```python
from build123d import *

# Parameters (mm, degrees)
SKETCH1_W           = 80
SKETCH1_H           = 80
BOSS_EXTRUDE3_DEPTH = 2
BOSS_EXTRUDE5_DEPTH = 77.35
CUT_EXTRUDE1_REACH  = 58.918
SKETCH7_W           = 64.6
SKETCH7_H           = 77
SKETCH5_W           = 80
SKETCH5_H           = 80
SKETCH5_W_2         = 77
SKETCH5_H_2         = 77
BOSS_EXTRUDE6_DEPTH = 44.8
SKETCH8_W           = 80
SKETCH8_H           = 80
BOSS_EXTRUDE7_DEPTH = 1.5


with BuildPart() as part:
    # Sketch1 → Boss-Extrude3 (new body)
    with BuildSketch(Plane(origin=(0, 0, 0), x_dir=(1, 0, 0), z_dir=(0, 1, 0))):
        Rectangle(SKETCH1_W, SKETCH1_H)
    extrude(amount=-BOSS_EXTRUDE3_DEPTH)

    # Sketch3 → Boss-Extrude5 (add)
    with BuildSketch(Plane.XY.offset(40)):
        Polygon((-32.3, -2), (-34.8, -2), (-34.8, -4.3), (-37.3, -4.3), (-37.3, -6.3), (-32.3, -6.3), align=None)
        Polygon((32.3, -6.3), (37.3, -6.3), (37.3, -4.3), (34.8, -4.3), (34.8, -2), (32.3, -2), align=None)
    extrude(amount=-BOSS_EXTRUDE5_DEPTH)

    # Sketch7 → Cut-Extrude1 (cut, up to next)
    with BuildSketch(Plane(origin=(0, 0, 0), x_dir=(1, 0, 0), z_dir=(0, 1, 0)), mode=Mode.PRIVATE) as cut_extrude1_sk1:
        Rectangle(SKETCH7_W, SKETCH7_H)
    cut_extrude1_tool1 = extrude(cut_extrude1_sk1.sketch, amount=-CUT_EXTRUDE1_REACH, mode=Mode.PRIVATE) & part.part
    add(cut_extrude1_tool1.solids().sort_by_distance((0, 0, 0))[0], mode=Mode.SUBTRACT)

    # Sketch5 → Boss-Extrude6 (add)
    with BuildSketch(Plane(origin=(0, 0, 0), x_dir=(1, 0, 0), z_dir=(0, 1, 0))):
        Rectangle(SKETCH5_W, SKETCH5_H)
        Rectangle(SKETCH5_W_2, SKETCH5_H_2, mode=Mode.SUBTRACT)
    extrude(amount=BOSS_EXTRUDE6_DEPTH)

    # Sketch8 → Boss-Extrude7 (add)
    with BuildSketch(Plane(origin=(0, 44.8, 0), x_dir=(1, 0, 0), z_dir=(0, 1, 0))):
        Rectangle(SKETCH8_W, SKETCH8_H)
    extrude(amount=-BOSS_EXTRUDE7_DEPTH)


solid = part.part
```
Can you work these out from the model? Positions are in its coordinate system, mm. A direction names the side the tool comes from. Coordinates: 2 decimals unless noted, no trailing zeros. Loops run counter-clockwise (first coordinate to the right, second up) from the corner with the lowest first, then second, coordinate; pieces in that order, holes last. Notation, with made-up numbers: M 25,22.25 L 63,22.25 A33 ccw 63,50.25 Z; hole C 35.5,17.25 d4. An arc over 180 degrees is marked long. Put each result on its own line as item: value. Start each with the question number.
(1) Imagine slicing it at C-C on z = 24. List the corners of the cut face in (x, y) for me.
(2) Which directions (+Z, -Z, +X, -X, +Y, -Y) give clear straight access to the entire face, cutting with the end or side of a thin tool? Please do faces 4 (the face through (34, -5, -37.35)), 5 (the face through (37.3, -5, 2)), 6 (the face through (32.3, -3, 1)), 7 (the face through (-36, -4.3, 2)), 8 (the face through (-1, 43.3, -1)).
(3) We'd pull the mould along Y, two halves only. Please class faces 1 (the face through (-32.3, -3, 1)), 2 (the face through (-1, 20, 38.5)), 3 (the face through (-1, 44.8, -1)): +Y half, -Y half, draft (parallel to the pull), parting line (faces both ways), or undercut.
(4) I need wall thicknesses on probe 1 along X at (y, z) = (13, -5.5); probe 2 along X at (y, z) = (-4, -14). Which ranges of each line are inside material? Lowest first, please.
(5) Will these pins go through, and if not, where does the flat tip stop? pin 1 Ø1.8 at (y, z) = (-3.5, 12.5) entering from +X; pin 2 Ø12 at (x, z) = (25, 13) entering from -Y; pin 3 Ø1.3 at (x, y) = (34, -3.5) entering from -Z; pin 4 Ø1.2 at (y, z) = (-2.5, 2) entering from -X.
(6) Imagine slicing it at A-A on y = 27. List the corners of the cut face in (x, z) for me.
(7) Imagine slicing it at B-B on x = 19. List the corners of the cut face in (y, z) for me, and give its area (3 significant figures).
Worked answers:
1. outline: M -40,-2 L -34.8,-2 L -34.8,-4.3 L -37.3,-4.3 L -37.3,-6.3 L -32.3,-6.3 L -32.3,0 L -38.5,0 L -38.5,43.3 L 38.5,43.3 L 38.5,0 L 32.3,0 L 32.3,-6.3 L 37.3,-6.3 L 37.3,-4.3 L 34.8,-4.3 L 34.8,-2 L 40,-2 L 40,44.8 L -40,44.8 Z
2. face 4: -Z, +X, -X, -Y
2. face 5: +Z, -Z, +X, -Y
2. face 6: -Y
2. face 7: +Z, -Z, -X
2. face 8: none
3. face 1: draft
3. face 2: undercut
3. face 3: +Y half
4. probe 1: x = -40 to -38.5, 38.5 to 40
4. probe 2: x = -34.8 to -32.3, 32.3 to 34.8
5. pin 1: stops at x = 37.3
5. pin 2: stops at y = 43.3
5. pin 3: stops at z = -37.35
5. pin 4: stops at x = -40
6. outline: M -40,-40 L 40,-40 L 40,40 L -40,40 Z; hole M -38.5,-38.5 L 38.5,-38.5 L 38.5,38.5 L -38.5,38.5 Z
7. outline: M -2,-40 L 44.8,-40 L 44.8,40 L -2,40 L -2,38.5 L 43.3,38.5 L 43.3,-38.5 L -2,-38.5 Z
7. area: 256 mm2
